```python
from build123d import *

# Parameters (mm, degrees)
F0_R     = 2.38125
F1_DEPTH = 7.366
F3_D     = 3.6576
F4_SIZE2 = 0.254
F4_SIZE  = 0.254


with BuildPart() as f1:
    # F0 (on Front) → F1 (new body)
    with BuildSketch(Plane.XZ):
        Circle(F0_R)
    extrude(amount=F1_DEPTH)

    # F3 (through all)
    with Locations(Plane.XZ.offset(7.366)):
        with Locations((0, 0)):
            Hole(F3_D / 2)

    # F4
    f4_edges = [f1.edges().sort_by_distance(p)[0] for p in [
        (-2.38125, -7.366, 0),
        (-2.38125, 0, 0),
    ]]
    chamfer(f4_edges, length=F4_SIZE, length2=F4_SIZE2)


solid = f1.part
```
Verification items for the finished model (mm, model axes). Round coordinates to 2 decimals unless told otherwise and drop trailing zeros. Write each loop counter-clockwise with the first axis right and the second up, starting at its lowest first coordinate (ties: lowest second). Pieces come first, ordered by that corner, then holes.
1. Draft check along Z on faces 1 (the cylindrical face through (1.451, -3.631, -1.113)), 2 (the cylindrical face through (-1.89, -3.63, -1.45)). Enter one of: +Z half, -Z half, draft (parallel to the pull), parting line (faces both ways), or undercut.
2. Scan lines: L1, parallel to Z at x = 0, y = -5.25; L2, parallel to Z at x = 1.5, y = -1; L3, parallel to X at y = -0.75, z = 0.8. Record each from-to range of solid material in increasing order.
3. Section check C-C on y = -3.75. Enter the section's corners in (x, z).
4. Section check A-A on z = 0. Enter the section's corners in (x, y), plus the area to 3 significant figures.
5. Section check B-B on x = 0. Enter the section's corners in (y, z).
Answer:
1. face 1: undercut
1. face 2: parting line
2. L1: z = -2.38 to -1.83, 1.83 to 2.38
2. L2: z = -1.85 to -1.05, 1.05 to 1.85
2. L3: x = -2.24 to -1.64, 1.64 to 2.24
3. outline: circle Ø4.76 at (0, 0); hole circle Ø3.66 at (0, 0)
4. outline: (-2.38, -7.11) - (-2.13, -7.37) - (-1.83, -7.37) - (-1.83, 0) - (-2.13, 0) - (-2.38, -0.25) - close; (1.83, -7.37) - (2.13, -7.37) - (2.38, -7.11) - (2.38, -0.25) - (2.13, 0) - (1.83, 0) - close
4. area: 8.01 mm2
5. outline: (-7.37, -2.13) - (-7.11, -2.38) - (-0.25, -2.38) - (0, -2.13) - (0, -1.83) - (-7.37, -1.83) - close; (-7.37, 1.83) - (0, 1.83) - (0, 2.13) - (-0.25, 2.38) - (-7.11, 2.38) - (-7.37, 2.13) - close
